Input: dimensioned drawing with shaded views. Units: mm. Origin: part minimum x, y, z. A direction names the side the tool comes from. Round coordinates to 2 decimals unless told otherwise and drop trailing zeros. Loops run counter-clockwise (first coordinate to the right, second up) from the corner with the lowest first, then second, coordinate; pieces in that order, holes last. Notation, with made-up numbers: M -10,37.25 L 25,37.25 A21 ccw 25,51.25 Z; hole C 76.5,51.5 d2. An arc over 180 degrees is marked long. One line per item, written item: value.
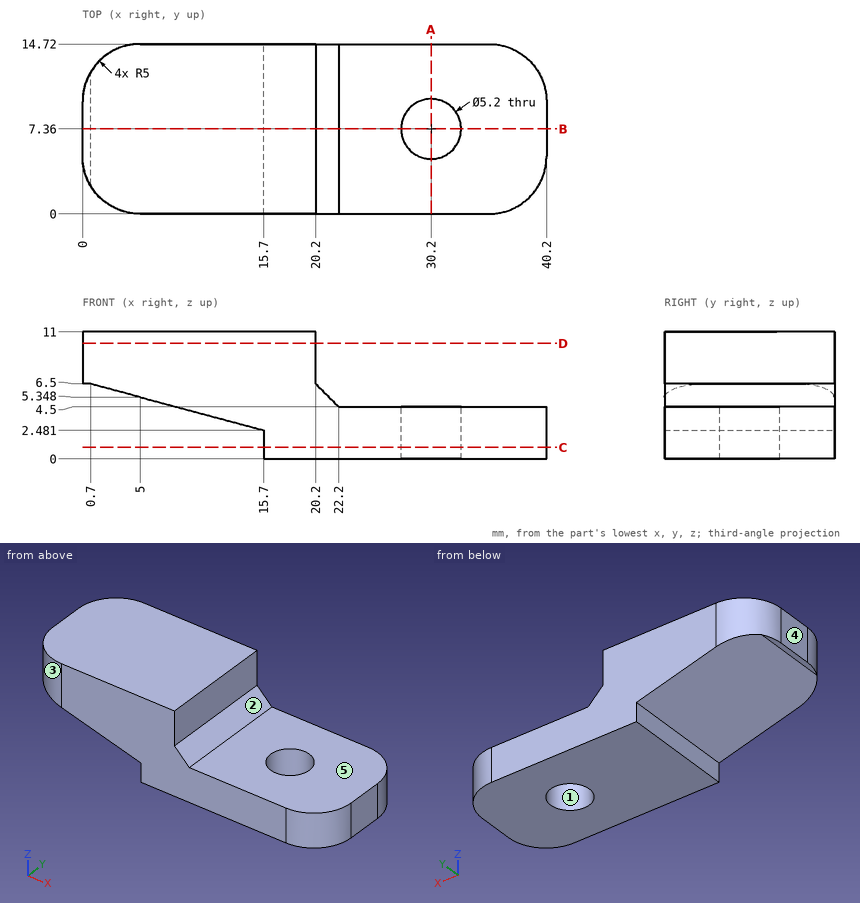
1. Ray query, line 1 (Y direction, x = 30.2, z = 1.6); line 2 (Z direction, x = 26, y = 6); line 3 (X direction, y = 8.5, z = 10). Return the intervals inside material, ascending. Write a range as [from, to].
Report:
line 1: y = [0, 4.76], [9.96, 14.72]
line 2: z = [0, 4.5]
line 3: x = [0, 20.2]
2. Pull-direction query (Y, two-part tool) for the marked faces 1, 2 and 3; classes: released by +Y, released by -Y, zero draft, split by the parting line, or undercut.
Report:
face 1: undercut
face 2: zero draft
face 3: released by -Y
3. Section query B-B (y = 7.36). Return the cut outline in (x, z), and give its area (3 significant figures).
Report:
outline: M 0,6.5 L 0.7,6.5 L 15.7,2.48 L 15.7,0 L 27.6,0 L 27.6,4.5 L 22.2,4.5 L 20.2,6.5 L 20.2,11 L 0,11 Z; M 32.8,0 L 40.2,0 L 40.2,4.5 L 32.8,4.5 Z
area: 219 mm2
4. Section query D-D (z = 10). Return the cut outline in (x, y), and give its area (3 significant figures).
Report:
outline: M 0,5 A5 ccw 5,0 L 20.2,0 L 20.2,14.72 L 5,14.72 A5 ccw 0,9.72 Z
area: 287 mm2
5. Section query C-C (z = 1). Return the cut outline in (x, y), and give its area (3 significant figures).
Report:
outline: M 15.7,0 L 35.2,0 A5 ccw 40.2,5 L 40.2,9.72 A5 ccw 35.2,14.72 L 15.7,14.72 Z; hole C 30.2,7.36 d5.2
area: 329 mm2
6. Section query A-A (x = 30.2). Return the cut outline in (y, z).
Report:
outline: M 0,0 L 4.76,0 L 4.76,4.5 L 0,4.5 Z; M 9.96,0 L 14.72,0 L 14.72,4.5 L 9.96,4.5 Z
7. Reachability of the marked faces 4 and 5 from +Z, -Z, +X, -X, +Y, -Y: full face, straight path, thin tool, end or side. Return the list, or none.
Report:
face 4: +Z, -Z, -X, +Y, -Y
face 5: +Z, +X, +Y, -Y
8. Pin query (flat end, axial travel): pin 1 (5 mm diameter, centred on x = 34, y = 12, fed in from +Z); pin 2 (4 mm diameter, centred on x = 30.2, y = 7.36, fed in from +Z); pin 3 (1.3 mm diameter, centred on y = 6.5, z = 8, fed in from +X). Return the tip coordinate at first contact, or that it passes through.
Report:
pin 1: stops at z = 4.5
pin 2: passes through
pin 3: stops at x = 20.2
